The model under review builds one solid part; all positions refer to its coordinate system, in mm. A direction names the side the tool comes from. Round coordinates to 2 decimals unless told otherwise and drop trailing zeros. Write each loop counter-clockwise with the first axis right and the second up, starting at its lowest first coordinate (ties: lowest second). Pieces come first, ordered by that corner, then holes. Notation, with made-up numbers: (72.25, 34.5) -> (114.25, 34.5) arc R24 ccw to (114.25, 66.5) -> close; hole circle Ø8 at (6, -29.75). An arc over 180 degrees is marked (long way). Answer as a JSON object with one key per item and string values. Group by question number.
1) Machinability: for faces 4 (the flat face through (92, 1, -25)), 5 (the cylindrical face through (8.8, 1.5, -1.6)), 6 (the cylindrical face through (75.178, 1.479, -23.384)), which of the approach directions +Z, -Z, +X, -X, +Y, -Y give a long, thin tool a straight path to every point of the face, cutting with its end or side? Answer none if there is none.
2) We need section C-C, the plane x = 46.5. Write out the cut boundary in (y, z).
3) Insertion check: pin 1 Ø1.5 at (x, y) = (35, 1.5) entering from +Z. The pin has a flat end and moves straight along its axis. Give the tip position at first contact, or say it passes through.
4) To check wall thickness, follow probe 1 along Z at (x, y) = (54, 0.75); probe 2 along X at (y, z) = (2.2, -2.25); probe 3 along X at (y, z) = (0.7, -2.5). State the ranges of each line that lie inside material, in increasing order. Write a range as [from, to].
5) We need section A-A, the plane z = -21. Write out the cut boundary in (x, y).
6) Mouldability with a two-part tool opening along X and no side actions: class faces 1 (the flat face through (92, 1, 0)), 2 (the cylindrical face through (63.33, 1.479, -16.356)), 3 (the flat face through (99.51, 1, -13)) as pulls with the +X half, pulls with the -X half, needs draft (parallel to the pull), parting line crosses it, or undercut.
7) We need section B-B, the plane y = 0.9. Write out the cut boundary in (x, z).
8) We need section D-D, the plane z = -3.75. Write out the cut boundary in (x, y).
from build123d import *

# Parameters (mm, degrees)
BOSS_EXTRUDE1_DEPTH = 3


with BuildPart() as part:
    # Sketch3 → Boss-Extrude1 (new body)
    with BuildSketch(Plane(origin=(0, 0, 0), x_dir=(1, 0, 0), z_dir=(0, 1, 0))):
        with BuildLine():
            Line((0, 0), (-15.490197962, 0))
            Line((-15.490197962, 0), (-15.490197962, 25))
            Line((-15.490197962, 25), (0, 25))
            ThreePointArc((0, 25), (8.724780506, 23.428149844), (16.352437204, 18.91025641))
            ThreePointArc((16.352437204, 18.91025641), (20.623924954, 16.380236087), (25.509802038, 15.5))
            Line((25.509802038, 15.5), (58.509802038, 15.5))
            ThreePointArc((58.509802038, 15.5), (63.395679121, 16.380236087), (67.667166872, 18.91025641))
            ThreePointArc((67.667166872, 18.91025641), (75.29482357, 23.428149844), (84.019604075, 25))
            Line((84.019604075, 25), (99.509802038, 25))
            Line((99.509802038, 25), (99.509802038, 0))
            Line((99.509802038, 0), (84.019604075, 0))
            ThreePointArc((84.019604075, 0), (75.29482357, 1.571850156), (67.667166872, 6.08974359))
            ThreePointArc((67.667166872, 6.08974359), (63.395679121, 8.619763913), (58.509802038, 9.5))
            Line((58.509802038, 9.5), (25.509802038, 9.5))
            ThreePointArc((25.509802038, 9.5), (20.623924954, 8.619763913), (16.352437204, 6.08974359))
            ThreePointArc((16.352437204, 6.08974359), (8.724780506, 1.571850156), (0, 0))
        make_face()
    extrude(amount=BOSS_EXTRUDE1_DEPTH)


solid = part.part
Here are the results:
{
 "1": {"face 4": "-Z, +X, -X, +Y, -Y", "face 5": "+Z, +Y, -Y", "face 6": "-Z, +Y, -Y"},
 "2": {"outline": "(0, -15.5) -> (3, -15.5) -> (3, -9.5) -> (0, -9.5) -> close"},
 "3": {"pin 1": "stops at z = -9.5"},
 "4": {"probe 1": "z = [-15.5, -9.5]", "probe 2": "x = [-15.49, 10.37], [73.65, 99.51]", "probe 3": "x = [-15.49, 10.9], [73.12, 99.51]"},
 "5": {"outline": "(-15.49, 0) -> (13.56, 0) -> (13.56, 3) -> (-15.49, 3) -> close; (70.45, 0) -> (99.51, 0) -> (99.51, 3) -> (70.45, 3) -> close"},
 "6": {"face 1": "needs draft", "face 2": "undercut", "face 3": "pulls with the +X half"},
 "7": {"outline": "(-15.49, -25) -> (0, -25) arc R25 ccw to (16.35, -18.91) arc R14 cw to (25.51, -15.5) -> (58.51, -15.5) arc R14 cw to (67.67, -18.91) arc R25 ccw to (84.02, -25) -> (99.51, -25) -> (99.51, 0) -> (84.02, 0) arc R25 ccw to (67.67, -6.09) arc R14 cw to (58.51, -9.5) -> (25.51, -9.5) arc R14 cw to (16.35, -6.09) arc R25 ccw to (0, 0) -> (-15.49, 0) -> close"},
 "8": {"outline": "(-15.49, 0) -> (13.17, 0) -> (13.17, 3) -> (-15.49, 3) -> close; (70.85, 0) -> (99.51, 0) -> (99.51, 3) -> (70.85, 3) -> close"}
}
